```python
from build123d import *

# Parameters (mm, degrees)
SKETCH3_W          = 60
SKETCH3_H          = 1
SKETCH4_W          = 6.07081849
SKETCH4_H          = 35
CUT_EXTRUDE1_DEPTH = 62.929395282
SKETCH5_R          = 2
CUT_EXTRUDE2_DEPTH = 62.85668921


with BuildPart() as part:
    # Sweep1: sweep along a path in Sketch1
    with BuildLine(Plane.XY) as sweep1_path:
        Line((0, 0), (12, 0))
        ThreePointArc((12, 0), (13.315747679, 4.62574882), (9.762440739, 1.384953564))
    # Sketch3 → Sweep1 (sweep)
    with BuildSketch(Plane(origin=(0, 0, 0), x_dir=(0, 0, -1), z_dir=(1, 0, 0))):
        with Locations((-30, 0.5)):
            Rectangle(SKETCH3_W, SKETCH3_H)
    sweep(path=sweep1_path.line)

    # Sketch4 → Cut-Extrude1 (cut, through all)
    with BuildSketch(Plane(origin=(0, 0, 0), x_dir=(-1, 0, 0), z_dir=(0, -1, 0))):
        with Locations((-12, -30)):
            Rectangle(SKETCH4_W, SKETCH4_H)
    extrude(amount=-CUT_EXTRUDE1_DEPTH, mode=Mode.SUBTRACT)

    # Sketch5 → Cut-Extrude2 (cut, through all)
    with BuildSketch(Plane(origin=(0, 1, 0), x_dir=(1, 0, 0), z_dir=(0, 1, 0))):
        with Locations(Location((4.212926144, -5.917287591, 0), (0, 0, 270))):
            Circle(SKETCH5_R)
        with Locations(Location((4.212926144, -54.082712409, 0), (0, 0, 90))):
            Circle(SKETCH5_R)
        with Locations(Location((4.212926144, -30, 0), (0, 0, 270))):
            Circle(SKETCH5_R)
    extrude(amount=-CUT_EXTRUDE2_DEPTH, mode=Mode.SUBTRACT)


solid = part.part
```
For this review, take the finished solid that the model builds, in its own axes (mm). A direction names the side the tool comes from. Round coordinates to 2 decimals unless told otherwise and drop trailing zeros. Write each loop counter-clockwise with the first axis right and the second up, starting at its lowest first coordinate (ties: lowest second). Pieces come first, ordered by that corner, then holes. Notation, with made-up numbers: (53, 13.25) - (97, 13.25) arc R19 cw to (97, 43.25) - close; hole circle Ø11 at (61, 43.5). An arc over 180 degrees is marked (long way). Write each question's results on one line, items separated by ' | '.
Item 1: To check wall thickness, follow line 1 along X through (y, z) = (2.5, 50.25); line 2 along Y through (x, z) = (12, 52.5); line 3 along Z through (x, y) = (13.25, 1). State the ranges of each line that lie inside material, in increasing order. Write a range as from..to.
Calculated:
line 1: x = 9.5..10.5, 13.5..14.5 | line 2: y = 0..1, 4..5 | line 3: z = 0..12.5, 47.5..60
Item 2: Take a section at B-B on y = 2.5. State the section outline as (x, z) points.
Calculated:
outline: (9.5, 0) - (10.5, 0) - (10.5, 12.5) - (9.5, 12.5) - close; (9.5, 47.5) - (10.5, 47.5) - (10.5, 60) - (9.5, 60) - close; (13.5, 0) - (14.5, 0) - (14.5, 12.5) - (13.5, 12.5) - close; (13.5, 47.5) - (14.5, 47.5) - (14.5, 60) - (13.5, 60) - close
Item 3: For pin 1 (5 mm diameter, centred on x = 7, z = 43, fed in from +Y); pin 2 (3 mm diameter, centred on y = 0.5, z = 13, fed in from +X); pin 3 (0.5 mm diameter, centred on y = 0.5, z = 33, fed in from +X), all flat-tipped, find the tip position at first contact; note any pin that passes through.
Calculated:
pin 1: stops at y = 1 | pin 2: stops at x = 14.43 | pin 3: stops at x = 8.96
Item 4: Take a section at A-A on z = 30. State the section outline as (x, y) points.
Calculated:
outline: (0, 0) - (2.21, 0) - (2.21, 1) - (0, 1) - close; (6.21, 0) - (8.96, 0) - (8.96, 1) - (6.21, 1) - close
Item 5: Take a section at D-D on x = 7. State the section outline as (y, z) points.
Calculated:
outline: (0, 0) - (1, 0) - (1, 60) - (0, 60) - close
Item 6: Take a section at C-C on z = 49.5. State the section outline as (x, y) points, then the cut area to 3 significant figures.
Calculated:
outline: (0, 0) - (12, 0) arc R2.5 ccw (long way) to (9.76, 1.38) - (10.66, 1.83) arc R1.5 cw (long way) to (12, 1) - (0, 1) - close | area: 22.3 mm^2
Item 7: For faces 1 (the face through (12.835, 3.746, 53.838)), 2 (the face through (13, 1, 47.5)), list the 3-axis set-ups (+Z, -Z, +X, -X, +Y, -Y) from which the entire face can be reached by the end or side of a thin tool; tool diameter is ignored.
Calculated:
face 1: +Z, -Z | face 2: +X, +Y, -Y
Item 8: Draft analysis for pull direction X (two halves, no side actions). For faces 3 (the face through (7, 1, 30)), 4 (the face through (0, 0.5, 29.6)), 5 (the face through (12.835, 3.746, 6.337)), state which applies: pulls with the +X half, pulls with the -X half, needs draft (parallel to the pull), parting line crosses it, or undercut.
Calculated:
face 3: needs draft | face 4: pulls with the -X half | face 5: undercut
